Here's how the part is built. I have some questions about the finished solid (model axes, mm). A direction names the side the tool comes from. Round coordinates to 2 decimals unless told otherwise and drop trailing zeros. Order: outer loops, then holes, each group sorted by start corner. A loop starts at its lowest first (then second) coordinate and runs counter-clockwise, first axis right, second up. Notation, with made-up numbers: (21, 36) - (39, 36) arc R26 ccw to (39, 71) - close; hole circle Ø8 at (8.5, 59.25). An arc over 180 degrees is marked (long way). One line per item, written item: value.
from build123d import *

# Parameters (mm, degrees)
SKETCH1_R           = 9.525
BOSS_EXTRUDE1_DEPTH = 7.9375
SKETCH2_R           = 9.525
BOSS_EXTRUDE2_DEPTH = 4.7625
SKETCH3_R           = 11.1125
BOSS_EXTRUDE3_DEPTH = 3.175
FILLET1_R           = 0.635
FILLET3_R           = 0.635
CHAMFER1_SIZE       = 0.635


with BuildPart() as part:
    # Sketch1 → Boss-Extrude1 (new body)
    with BuildSketch(Plane(origin=(0, 0, 0), x_dir=(1, 0, 0), z_dir=(0, 1, 0))):
        with Locations(Location((0, 0, 0), (0, 0, 270))):
            Circle(SKETCH1_R)
        Polygon((5.865878735, 0), (2.932939367, 5.08), (-2.932939367, 5.08), (-5.865878735, 0), (-2.932939367, -5.08), (2.932939367, -5.08), align=None, mode=Mode.SUBTRACT)
    extrude(amount=BOSS_EXTRUDE1_DEPTH)

    # Sketch2 → Boss-Extrude2 (add)
    with BuildSketch(Plane(origin=(0, 7.9375, 0), x_dir=(1, 0, 0), z_dir=(0, 1, 0))):
        with Locations(Location((0, 0, 0), (0, 0, 270))):
            Circle(SKETCH2_R)
        Polygon((-2.932939367, 5.08), (-5.865878735, 0), (-2.932939367, -5.08), (2.932939367, -5.08), (5.865878735, 0), (2.932939367, 5.08), align=None, mode=Mode.SUBTRACT)
    extrude(amount=BOSS_EXTRUDE2_DEPTH)

    # Sketch3 → Boss-Extrude3 (add)
    with BuildSketch(Plane.XZ):
        with Locations(Location((0, 0, 0), (0, 0, 270))):
            Circle(SKETCH3_R)
        Polygon((-2.932939367, 5.08), (2.932939367, 5.08), (5.865878735, 0), (2.932939367, -5.08), (-2.932939367, -5.08), (-5.865878735, 0), align=None, mode=Mode.SUBTRACT)
    extrude(amount=BOSS_EXTRUDE3_DEPTH)

    # Fillet1
    fillet1_edges = [part.edges().sort_by_distance(p)[0] for p in [
        (0, 0, -9.525),
        (0, 0, 11.1125),
    ]]
    fillet(fillet1_edges, radius=FILLET1_R)

    # Fillet3
    fillet3_edges = [part.edges().sort_by_distance(p)[0] for p in [
        (0, 12.7, -9.525),
        (0, 12.7, -5.08),
        (-4.399409051, 12.7, -2.54),
        (-4.399409051, 12.7, 2.54),
        (0, 12.7, 5.08),
        (4.399409051, 12.7, 2.54),
        (4.399409051, 12.7, -2.54),
    ]]
    fillet(fillet3_edges, radius=FILLET3_R)

    # Chamfer1
    chamfer1_edges = [part.edges().sort_by_distance(p)[0] for p in [
        (0, -3.175, 11.1125),
        (-4.399409051, -3.175, 2.54),
        (-4.399409051, -3.175, -2.54),
        (0, -3.175, -5.08),
        (4.399409051, -3.175, -2.54),
        (4.399409051, -3.175, 2.54),
        (0, -3.175, 5.08),
    ]]
    chamfer(chamfer1_edges, length=CHAMFER1_SIZE)


solid = part.part
Q1. Which directions (+Z, -Z, +X, -X, +Y, -Y) give clear straight access to the entire face, cutting with the end or side of a thin tool? Please do faces 1 (the flat face through (4.42, 4.865, -2.504)), 2 (the flat face through (-4.7, -2.86, 2.66)), 3 (the cylindrical face through (4.58, 12.51, 2.59)), 4 (the flat face through (-5, -3.175, -5)).
Results list:
face 1: +Y, -Y
face 2: -Y
face 3: +Y
face 4: +Z, -Z, +X, -X, -Y
Q2. We'd pull the mould along X, two halves only. Please class faces 5 (the cylindrical face through (-4.58, 12.51, -2.59)), 6 (the flat face through (0, 12.7, 6)), 7 (the cylindrical face through (-5.796, 6.27, -7.559)): released by +X, released by -X, zero draft, split by the parting line, or undercut.
Results list:
face 5: undercut
face 6: zero draft
face 7: split by the parting line
Q3. Will these pins go through, and if not, where does the flat tip stop? pin 1 (4 mm diameter, centred on y = 5, z = 1.5, fed in from +X) (3 decimals); pin 2 (4 mm diameter, centred on y = 9.5, z = 6, fed in from +X); pin 3 (6.5 mm diameter, centred on x = 0.5, y = 8.5, fed in from +Z) (3 decimals); pin 4 (4 mm diameter, centred on x = -3.5, z = 4, fed in from -Y) (3 decimals).
Results list:
pin 1: x = 9.525
pin 2: x = 8.64
pin 3: z = 9.525
pin 4: y = -3.175
Q4. If we section it at B-B, the plane y = 10.5: Please give me the cut outline in (x, z) (3 decimals), then the cut area to 3 significant figures.
Results list:
outline: circle Ø19.05 at (0, 0); hole (-5.866, 0) - (-2.933, -5.08) - (2.933, -5.08) - (5.866, 0) - (2.933, 5.08) - (-2.933, 5.08) - close
area: 196 mm²
Q5. If I drill on line 1 along Z through (x, y) = (-2.25, 3.5); line 2 along X through (y, z) = (11.5, 2.5); line 3 along X through (y, z) = (0.5, 0.5), over which ranges is the centre line in solid material (lowest first)?
Results list:
line 1: -9.26 to -5.08, 5.08 to 9.26
line 2: -9.19 to -4.42, 4.42 to 9.19
line 3: -9.53 to -5.58, 5.58 to 9.53
